Here's how the part is built. I have some questions about the finished solid (model axes, mm). Face numbers are marked on the shaded views. A direction names the side the tool comes from. Coordinates: 2 decimals unless noted, no trailing zeros. Write each loop counter-clockwise with the first axis right and the second up, starting at its lowest first coordinate (ties: lowest second). Pieces come first, ordered by that corner, then holes.
Item 1: If we section it at C-C (y = 9): Please give me the cut outline in (x, z).
Item 2: I'm going to push flat-ended pins straight in: pin 1 Ø1.5 at (x, y) = (1.5, 14.5) entering from +Z; pin 2 Ø0.8 at (x, z) = (0, -7) entering from -Y; pin 3 Ø5 at (y, z) = (3, -6) entering from -X. Where does each tip first touch, or does it pass through?
Item 3: We'd pull the mould along Z, two halves only. Please class the marked faces 1, 2 and 3: +Z half, -Z half, draft (parallel to the pull), parting line (faces both ways), or undercut.
Item 4: If we section it at B-B (x = 0): Please give me the cut outline in (y, z).
Item 5: If I drill on line 1 (Z direction, x = 0, y = 10.25); line 2 (Y direction, x = -1.5, z = 4), over which ranges is the centre line in solid material (lowest first)?
Item 6: If we section it at A-A (z = 0): Please give me the cut outline in (x, y).
Item 7: If we section it at D-D (x = 3.5): Please give me the cut outline in (y, z).
Item 8: For the marked faces 4 and 5, which set-ups out of +Z, -Z, +X, -X, +Y, -Y let a thin tool reach every point of the face, with its end or its side?
from build123d import *

# Parameters (mm, degrees)
SKETCH1_R           = 7.5
SKETCH1_R_2         = 3
BOSS_EXTRUDE1_DEPTH = 6
SKETCH2_R           = 7.5
SKETCH2_R_2         = 5.5
BOSS_EXTRUDE2_DEPTH = 10
CUT_EXTRUDE1_DEPTH  = 7


with BuildPart() as part:
    # Sketch1 → Boss-Extrude1 (new body)
    with BuildSketch(Plane(origin=(0, 0, 0), x_dir=(1, 0, 0), z_dir=(0, 1, 0))):
        with Locations(Location((0, 0, 0), (0, 0, 270))):
            Circle(SKETCH1_R)
        with Locations(Location((0, 0, 0), (0, 0, 270))):
            Circle(SKETCH1_R_2, mode=Mode.SUBTRACT)
    extrude(amount=BOSS_EXTRUDE1_DEPTH)

    # Sketch2 → Boss-Extrude2 (add)
    with BuildSketch(Plane(origin=(0, 6, 0), x_dir=(1, 0, 0), z_dir=(0, 1, 0))):
        with Locations(Location((0, 0, 0), (0, 0, 270))):
            Circle(SKETCH2_R)
        with Locations(Location((0, 0, 0), (0, 0, 270))):
            Circle(SKETCH2_R_2, mode=Mode.SUBTRACT)
    extrude(amount=BOSS_EXTRUDE2_DEPTH)

    # Sketch3 → Cut-Extrude1 (cut)
    with BuildSketch(Plane.XZ):
        with BuildLine():
            Line((-0.527362107, 10.532593193), (-0.527362107, 7.481436306))
            ThreePointArc((-0.527362107, 7.481436306), (0, 7.5), (0.527362107, 7.481436306))
            Line((0.527362107, 7.481436306), (0.527362107, 10.532593193))
            Line((0.527362107, 10.532593193), (-0.527362107, 10.532593193))
        make_face()
        with BuildLine():
            Line((-7.481436306, 0.527362107), (-10.459348456, 0.527362107))
            Line((-10.459348456, 0.527362107), (-10.459348456, -0.527362107))
            Line((-10.459348456, -0.527362107), (-7.481436306, -0.527362107))
            ThreePointArc((-7.481436306, -0.527362107), (-7.5, 0), (-7.481436306, 0.527362107))
        make_face()
        with BuildLine():
            ThreePointArc((0.527362107, 7.481436306), (0, 7.5), (-0.527362107, 7.481436306))
            Line((-0.527362107, 7.481436306), (-0.527362107, 2.953284478))
            ThreePointArc((-0.527362107, 2.953284478), (0, 3), (0.527362107, 2.953284478))
            Line((0.527362107, 2.953284478), (0.527362107, 7.481436306))
        make_face()
        with BuildLine():
            Line((-0.527362107, -2.953284478), (-0.527362107, -7.481436306))
            ThreePointArc((-0.527362107, -7.481436306), (0, -7.5), (0.527362107, -7.481436306))
            Line((0.527362107, -7.481436306), (0.527362107, -2.953284478))
            ThreePointArc((0.527362107, -2.953284478), (0, -3), (-0.527362107, -2.953284478))
        make_face()
        with BuildLine():
            Line((-2.953284478, 0.527362107), (-7.481436306, 0.527362107))
            ThreePointArc((-7.481436306, 0.527362107), (-7.5, 0), (-7.481436306, -0.527362107))
            Line((-7.481436306, -0.527362107), (-2.953284478, -0.527362107))
            ThreePointArc((-2.953284478, -0.527362107), (-3, 0), (-2.953284478, 0.527362107))
        make_face()
        with BuildLine():
            ThreePointArc((7.5, 0), (7.49535764, 0.263844368), (7.481436306, 0.527362107))
            Line((7.481436306, 0.527362107), (2.953284478, 0.527362107))
            ThreePointArc((2.953284478, 0.527362107), (2.988298298, 0.264713587), (3, 0))
            ThreePointArc((3, 0), (2.988298298, -0.264713587), (2.953284478, -0.527362107))
            Line((2.953284478, -0.527362107), (7.481436306, -0.527362107))
            ThreePointArc((7.481436306, -0.527362107), (7.49535764, -0.263844368), (7.5, 0))
        make_face()
    extrude(amount=-CUT_EXTRUDE1_DEPTH, mode=Mode.SUBTRACT)


solid = part.part
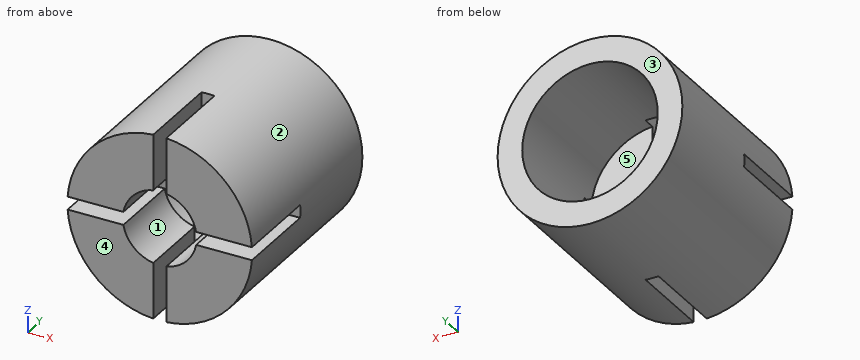
Answer list:
1. outline: circle Ø15 at (0, 0); hole circle Ø11 at (0, 0)
2. pin 1: stops at z = 7.46
2. pin 2: stops at y = 7
2. pin 3: stops at x = -6.63
3. face 1: undercut
3. face 2: parting line
3. face 3: draft
4. outline: (7, -7.5) - (16, -7.5) - (16, -5.5) - (7, -5.5) - close; (7, 5.5) - (16, 5.5) - (16, 7.5) - (7, 7.5) - close
5. line 1: z = -7.5 to -5.5, 5.5 to 7.5
5. line 2: y = 0 to 6
6. outline: (-7.5, 7) - (-5.5, 7) - (-5.5, 16) - (-7.5, 16) - close; (5.5, 7) - (7.5, 7) - (7.5, 16) - (5.5, 16) - close
7. outline: (0, -6.63) - (16, -6.63) - (16, -4.24) - (6, -4.24) - (6, -0.53) - (0, -0.53) - close; (0, 0.53) - (6, 0.53) - (6, 4.24) - (16, 4.24) - (16, 6.63) - (0, 6.63) - close
8. face 4: +Z, -Z, +X, -X, -Y
8. face 5: +Y
